```python
from build123d import *

# Parameters (mm, degrees)
SKETCH1_R           = 2.0828
BOSS_EXTRUDE1_DEPTH = 1.6
FILLET1_R           = 2.54
SKETCH3_R           = 2.0828
CUT_EXTRUDE1_DEPTH  = 79.362595117
SKETCH4_W           = 14.730000004
SKETCH4_H           = 1.456840112
BOSS_EXTRUDE2_DEPTH = 1.6
FILLET2_R           = 1


with BuildPart() as part:
    # Sketch1 → Boss-Extrude1 (new body)
    with BuildSketch(Plane.XY):
        with BuildLine():
            Line((7.903015948, 75.005885785), (22.633015952, 75.005885785))
            Line((22.633015952, 75.005885785), (22.633015952, 68.549399108))
            ThreePointArc((22.633015952, 68.549399108), (21.133015952, 64.505885785), (22.633015952, 60.462372462))
            Line((22.633015952, 60.462372462), (22.633015952, 45.943399108))
            ThreePointArc((22.633015952, 45.943399108), (21.133015952, 41.899885785), (22.633015952, 37.856372462))
            Line((22.633015952, 37.856372462), (22.633015952, 23.337399108))
            ThreePointArc((22.633015952, 23.337399108), (21.133015952, 19.293885785), (22.633015952, 15.250372462))
            Line((22.633015952, 15.250372462), (22.633015952, 0.731399108))
            ThreePointArc((22.633015952, 0.731399108), (21.133015952, -3.312114215), (22.633015952, -7.355627538))
            Line((22.633015952, -7.355627538), (22.633015952, -13.812114215))
            Line((22.633015952, -13.812114215), (7.903015948, -13.812114215))
            Line((7.903015948, -13.812114215), (7.903015948, -7.355627538))
            ThreePointArc((7.903015948, -7.355627538), (9.403015948, -3.312114215), (7.903015948, 0.731399108))
            Line((7.903015948, 0.731399108), (7.903015948, 15.250372462))
            ThreePointArc((7.903015948, 15.250372462), (9.403015948, 19.293885785), (7.903015948, 23.337399108))
            Line((7.903015948, 23.337399108), (7.903015948, 37.856372462))
            ThreePointArc((7.903015948, 37.856372462), (9.403015948, 41.899885785), (7.903015948, 45.943399108))
            Line((7.903015948, 45.943399108), (7.903015948, 60.462372462))
            ThreePointArc((7.903015948, 60.462372462), (9.403015948, 64.505885785), (7.903015948, 68.549399108))
            Line((7.903015948, 68.549399108), (7.903015948, 75.005885785))
        make_face()
        with Locations((15.26801595, 72.043125897)):
            Circle(SKETCH1_R, mode=Mode.SUBTRACT)
        with Locations(Location((15.26801595, -10.849354327, 0), (0, 0, 180))):
            Circle(SKETCH1_R, mode=Mode.SUBTRACT)
    extrude(amount=BOSS_EXTRUDE1_DEPTH)

    # Fillet1
    fillet1_edges = [part.edges().sort_by_distance(p)[0] for p in [
        (22.633015952, 68.549399108, 0.8),
        (22.633015952, 60.462372462, 0.8),
        (22.633015952, 45.943399108, 0.8),
        (22.633015952, 37.856372462, 0.8),
        (22.633015952, 23.337399108, 0.8),
        (22.633015952, 15.250372462, 0.8),
        (22.633015952, 0.731399108, 0.8),
        (22.633015952, -7.355627538, 0.8),
        (7.903015948, -7.355627538, 0.8),
        (7.903015948, 0.731399108, 0.8),
        (7.903015948, 15.250372462, 0.8),
        (7.903015948, 23.337399108, 0.8),
        (7.903015948, 37.856372462, 0.8),
        (7.903015948, 45.943399108, 0.8),
        (7.903015948, 60.462372462, 0.8),
        (7.903015948, 68.549399108, 0.8),
    ]]
    fillet(fillet1_edges, radius=FILLET1_R)

    # Sketch3 → Cut-Extrude1 (cut, through all)
    with BuildSketch(Plane.XY.offset(1.6)):
        with Locations((15.26801595, 30.596885785)):
            Circle(SKETCH3_R)
    extrude(amount=-CUT_EXTRUDE1_DEPTH, mode=Mode.SUBTRACT)

    # Sketch4 → Boss-Extrude2 (add, through all)
    with BuildSketch(Plane.XY.offset(1.6)):
        with Locations((15.26801595, -14.540534271)):
            Rectangle(SKETCH4_W, SKETCH4_H)
        with Locations((15.26801595, 75.734305841)):
            Rectangle(SKETCH4_W, SKETCH4_H)
    extrude(amount=-BOSS_EXTRUDE2_DEPTH)

    # Fillet2
    fillet2_edges = [part.edges().sort_by_distance(p)[0] for p in [
        (7.903015948, 76.462725897, 0.8),
        (22.633015952, 76.462725897, 0.8),
        (7.903015948, -15.268954327, 0.8),
        (22.633015952, -15.268954327, 0.8),
    ]]
    fillet(fillet2_edges, radius=FILLET2_R)


solid = part.part
```
Part model, mm, in its own coordinate system. A direction names the side the tool comes from. Coordinates: 2 decimals unless noted, no trailing zeros. Write each loop counter-clockwise with the first axis right and the second up, starting at its lowest first coordinate (ties: lowest second). Pieces come first, ordered by that corner, then holes.
Item 1: Slice it at C-C (z = 0.9). Count the separate pieces of the cut face and the enclosed holes in it, and give its area (3 significant figures).
Item 2: Slice it at A-A (x = 15). Write the cut outline in (y, z), and give its area (3 significant figures).
Item 3: Slice it at D-D (y = 20). Write the cut outline in (x, z), and give its area (3 significant figures).
Item 4: Which spindle directions (+Z, -Z, +X, -X, +Y, -Y) get a long thin tool onto all of the face, cutting with end or side? Do faces 4 (the face through (22.52, 15.15, 0.81)), 5 (the face through (22.633, 31, 1)), 6 (the face through (8, 46.1, 0.8)). Say none if no direction does.
Item 5: Mould opens along X. For faces 1 (the face through (21.133, 41.951, 0.789)), 2 (the face through (15, 74.11, 0.79)), 3 (the face through (8.02, 37.76, 0.81)) say: released by +X, released by -X, zero draft, split by the parting line, or undercut.
Item 6: Slice it at B-B (y = 71). Write the cut outline in (x, z).
Item 7: Probe line 1 (Y direction, x = 15.5, z = 1.45); line 2 (Y direction, x = 14.75, z = 1.2); line 3 (X direction, y = 41.5, z = 0.2). List the from-to ranges inside material, lowest first.
Results found:
1. separate pieces: 1
1. enclosed holes: 3
1. area: 1,240 mm2
2. outline: (-15.27, 0) - (-12.91, 0) - (-12.91, 1.6) - (-15.27, 1.6) - close; (-8.78, 0) - (28.53, 0) - (28.53, 1.6) - (-8.78, 1.6) - close; (32.66, 0) - (69.98, 0) - (69.98, 1.6) - (32.66, 1.6) - close; (74.11, 0) - (76.46, 0) - (76.46, 1.6) - (74.11, 1.6) - close
2. area: 127 mm2
3. outline: (9.36, 0) - (21.17, 0) - (21.17, 1.6) - (9.36, 1.6) - close
3. area: 18.9 mm2
4. face 4: +Z, -Z, +X
4. face 5: +Z, -Z, +X, +Y, -Y
4. face 6: +Z, -Z, -X
5. face 1: released by +X
5. face 2: undercut
5. face 3: released by -X
6. outline: (7.9, 0) - (13.47, 0) - (13.47, 1.6) - (7.9, 1.6) - close; (17.07, 0) - (22.63, 0) - (22.63, 1.6) - (17.07, 1.6) - close
7. line 1: y = -15.27 to -12.92, -8.78 to 28.53, 32.67 to 69.97, 74.11 to 76.46
7. line 2: y = -15.27 to -12.87, -8.83 to 28.58, 32.61 to 70.03, 74.06 to 76.46
7. line 3: x = 9.39 to 21.15
